Part model, mm, in its own coordinate system. Face numbers are marked on the shaded views. A direction names the side the tool comes from. Coordinates: 2 decimals unless noted, no trailing zeros. Loops run counter-clockwise (first coordinate to the right, second up) from the corner with the lowest first, then second, coordinate; pieces in that order, holes last. Notation, with made-up numbers: (41.25, 48.25) - (59.25, 48.25) arc R14 ccw to (59.25, 71.25) - close; hole circle Ø3 at (-14.75, 54). An arc over 180 degrees is marked (long way). Use a Markdown table: item, result. Add a question column.
1) Band-saw the part on D-D (z = 84.5). Give the cut face in (x, y).
2) Drop flat-ended pins along their axis: P1, Ø2, axis at y = 30, z = -24, coming from the -X side; P2, Ø1.5, axis at x = 14.5, y = 23.5, coming from the +Z side; P3, Ø1, axis at x = -64, y = 42.5, coming from the -Z side. Give the stop position or say it passes through.
3) Probe probe 1 along X at (y, z) = (46.5, 115); probe 2 along X at (y, z) = (2.45, -37.5); probe 3 along X at (y, z) = (3, 23.5). List the from-to ranges inside material, lowest first. Write a range as [from, to].
4) Tool access for the marked faces 1, 2, 3 and 4: list every direction of +Z, -Z, +X, -X, +Y, -Y with a clear straight run to the whole face (end or side of a thin tool).
5) Pull direction X, two halves, no side cores. Call the marked faces 5, 6, 7 and 8: +X half, -X half, draft (parallel to the pull), parting line (faces both ways), or undercut.
6) Band-saw the part on A-A (z = 43.5). Give the cut face in (x, y), plus the area to 3 significant figures.
7) Band-saw the part on B-B (y = 21.5). Give the cut face in (x, z).
8) Band-saw the part on C-C (x = -16). Give the cut face in (y, z).
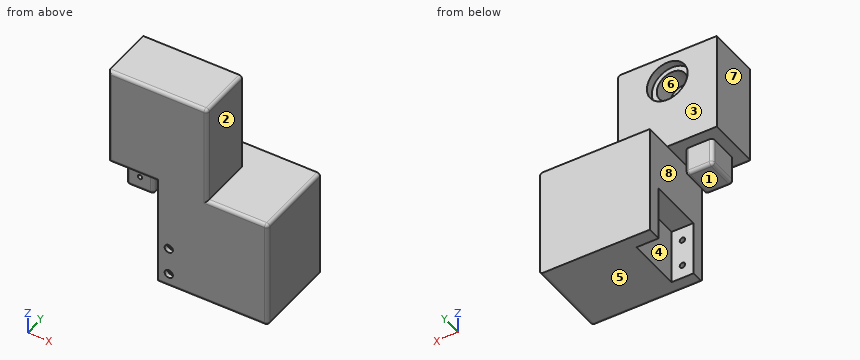
from build123d import *

# Parameters (mm, degrees)
SKETCH1_W           = 100
SKETCH1_H           = 100
BOSS_EXTRUDE1_DEPTH = 50
SKETCH8_W           = 90
SKETCH8_H           = 90
BOSS_EXTRUDE4_DEPTH = 50
SKETCH9_R           = 18.5
CUT_EXTRUDE1_DEPTH  = 7
SKETCH10_R          = 14
CUT_EXTRUDE2_DEPTH  = 25
SKETCH11_W          = 25
SKETCH11_H          = 30
BOSS_EXTRUDE5_DEPTH = 25
SKETCH12_W          = 100
SKETCH12_H          = 100
BOSS_EXTRUDE6_DEPTH = 25
SKETCH13_W          = 20
SKETCH13_H          = 50
CUT_EXTRUDE3_DEPTH  = 50
SKETCH14_R          = 2
CUT_EXTRUDE4_DEPTH  = 15
SKETCH15_R          = 2.5
CUT_EXTRUDE5_DEPTH  = 15
SKETCH16_R          = 3.75
CUT_EXTRUDE6_DEPTH  = 4
FILLET1_R           = 3


with BuildPart() as part:
    # Sketch1 → Boss-Extrude1 (new body)
    with BuildSketch(Plane(origin=(0, 0, 0), x_dir=(1, 0, 0), z_dir=(0, 1, 0))):
        Rectangle(SKETCH1_W, SKETCH1_H)
    extrude(amount=BOSS_EXTRUDE1_DEPTH)

    # Sketch8 → Boss-Extrude4 (add)
    with BuildSketch(Plane(origin=(0, 50, 0), x_dir=(1, 0, 0), z_dir=(0, 1, 0))):
        with Locations((-50, -95)):
            Rectangle(SKETCH8_W, SKETCH8_H)
    extrude(amount=-BOSS_EXTRUDE4_DEPTH)

    # Sketch9 → Cut-Extrude1 (cut)
    with BuildSketch(Plane(origin=(0, 50, 0), x_dir=(1, 0, 0), z_dir=(0, 1, 0))):
        with Locations(Location((-50, -115, 0), (0, 0, 270))):
            Circle(SKETCH9_R)
    extrude(amount=-CUT_EXTRUDE1_DEPTH, mode=Mode.SUBTRACT)

    # Sketch10 → Cut-Extrude2 (cut)
    with BuildSketch(Plane(origin=(0, 50, 0), x_dir=(1, 0, 0), z_dir=(0, 1, 0))):
        with Locations(Location((-50, -115, 0), (0, 0, 270))):
            Circle(SKETCH10_R)
    extrude(amount=-CUT_EXTRUDE2_DEPTH, mode=Mode.SUBTRACT)

    # Sketch11 → Boss-Extrude5 (add)
    with BuildSketch(Plane(origin=(0, 0, 50), x_dir=(-1, 0, 0), z_dir=(0, 0, -1))):
        with Locations((72.5, 25)):
            Rectangle(SKETCH11_W, SKETCH11_H)
    extrude(amount=BOSS_EXTRUDE5_DEPTH)

    # Sketch12 → Boss-Extrude6 (add)
    with BuildSketch(Plane(origin=(0, 50, 0), x_dir=(1, 0, 0), z_dir=(0, 1, 0))):
        Rectangle(SKETCH12_W, SKETCH12_H)
    extrude(amount=BOSS_EXTRUDE6_DEPTH)

    # Sketch13 → Cut-Extrude3 (cut)
    with BuildSketch(Plane(origin=(0, 0, -50), x_dir=(-1, 0, 0), z_dir=(0, 0, -1))):
        with Locations((40, 37.5)):
            Rectangle(SKETCH13_W, SKETCH13_H)
    extrude(amount=-CUT_EXTRUDE3_DEPTH, mode=Mode.SUBTRACT)

    # Sketch14 → Cut-Extrude4 (cut)
    with BuildSketch(Plane.XZ.offset(-10)):
        with Locations(Location((-72.5, 37.5, 0), (0, 0, 270))):
            Circle(SKETCH14_R)
    extrude(amount=-CUT_EXTRUDE4_DEPTH, mode=Mode.SUBTRACT)

    # Sketch15 → Cut-Extrude5 (cut)
    with BuildSketch(Plane.XZ):
        with Locations(Location((-40, -37.5, 0), (0, 0, 270))):
            Circle(SKETCH15_R)
        with Locations((-40, -12.5)):
            Circle(SKETCH15_R)
    extrude(amount=-CUT_EXTRUDE5_DEPTH, mode=Mode.SUBTRACT)

    # Sketch16 → Cut-Extrude6 (cut)
    with BuildSketch(Plane.XZ):
        with Locations(Location((-40, -37.5, 0), (0, 0, 270))):
            Circle(SKETCH16_R)
        with Locations(Location((-40, -12.5, 0), (0, 0, 90))):
            Circle(SKETCH16_R)
    extrude(amount=-CUT_EXTRUDE6_DEPTH, mode=Mode.SUBTRACT)

    # Fillet1
    fillet1_edges = [part.edges().sort_by_distance(p)[0] for p in [
        (22.5, 0, 50),
        (-5, 25, 140),
        (-5, 0, 95),
        (-50, 0, 140),
        (-95, 0, 95),
        (-72.5, 0, 50),
        (-85, 10, 37.5),
        (-85, 40, 37.5),
        (-60, 40, 37.5),
        (-60, 10, 37.5),
        (-85, 25, 25),
        (-72.5, 40, 25),
        (-60, 25, 25),
        (-72.5, 10, 25),
        (0, 0, -50),
        (50, 0, 0),
        (50, 37.5, 50),
        (50, 37.5, -50),
    ]]
    fillet(fillet1_edges, radius=FILLET1_R)


solid = part.part
Answer block:
| question | item | result |
|---|---|---|
| 1 | outline | (-95, 3) arc R3 ccw to (-92, 0) - (-8, 0) arc R3 ccw to (-5, 3) - (-5, 50) - (-95, 50) - close |
| 2 | P1 | x = -30 |
| 2 | P2 | z = 50 |
| 2 | P3 | z = 50 |
| 3 | probe 1 | [-95, -68.5], [-31.5, -5] |
| 3 | probe 2 | [-50, -43.75], [-36.25, 49.95] |
| 3 | probe 3 | [-50, 50] |
| 4 | face 1 | -Z, -X, +Y, -Y |
| 4 | face 2 | +Z, +X, +Y, -Y |
| 4 | face 3 | +Z, +X, -X, +Y |
| 4 | face 4 | -Z, -X |
| 5 | face 5 | draft |
| 5 | face 6 | undercut |
| 5 | face 7 | -X half |
| 5 | face 8 | undercut |
| 6 | outline | (-85, 13) arc R3 ccw to (-82, 10) - (-63, 10) arc R3 ccw to (-60, 13) - (-60, 37) arc R3 ccw to (-63, 40) - (-82, 40) arc R3 ccw to (-85, 37) - close; (-50, 0) - (47, 0) arc R3 ccw to (50, 3) - (50, 75) - (-50, 75) - close |
| 6 | area | 8,240 mm2 |
| 7 | outline | (-95, 50) - (-85, 50) - (-85, 28) arc R3 ccw to (-82, 25) - (-63, 25) arc R3 ccw to (-60, 28) - (-60, 50) - (-50, 50) - (-50, 0) - (-30, 0) - (-30, -50) - (47, -50) arc R3 ccw to (50, -47) - (50, 47) arc R3 ccw to (47, 50) - (-5, 50) - (-5, 137) arc R3 ccw to (-8, 140) - (-95, 140) - close; hole circle Ø4 at (-72.5, 37.5) |
| 8 | outline | (0, -47) arc R3 ccw to (3, -50) - (75, -50) - (75, 50) - (50, 50) - (50, 140) - (3, 140) arc R3 ccw to (0, 137) - close |
